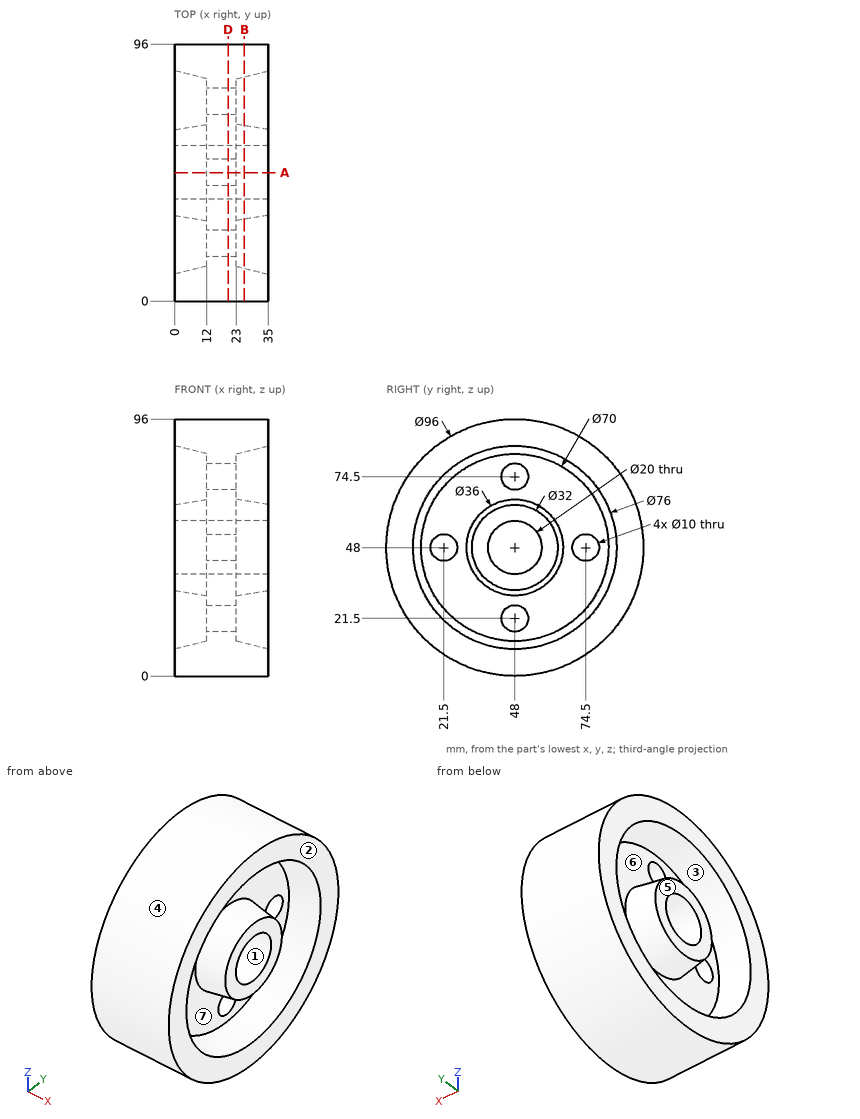
Input: dimensioned drawing with shaded views. Units: mm. Origin: part minimum x, y, z. A direction names the side the tool comes from. Coordinates: 2 decimals unless noted, no trailing zeros. Write each loop counter-clockwise with the first axis right and the second up, starting at its lowest first coordinate (ties: lowest second). Pieces come first, ordered by that corner, then holes. Notation, with made-up numbers: (30, -32) -> (84, -32) arc R22 ccw to (84, -4) -> close; hole circle Ø10 at (50, 29). An arc over 180 degrees is marked (long way). Return JSON: item names as keys, results as strings. Group by question number.
1) Ray query, line 1 along Y through (x, z) = (19, 48); line 2 along Z through (x, y) = (33, 52); line 3 along Z through (x, y) = (29, 46). Return the intervals inside material, ascending.
2) Section query D-D, the plane x = 20. Return loops of the section in (y, z).
3) Mould query, pull axis Y, two halves, no side actions, for the marked faces 1, 2, 3 and 4. Classes: +Y half, -Y half, draft (parallel to the pull), parting line (faces both ways), or undercut.
4) Section query A-A, the plane y = 48. State how many separate pieces and enclosed holes the cut face has, plus the area to 3 significant figures.
5) Contact query for flat-ended pins moving along their axis: P1, Ø1.5, axis at y = 45.5, z = 72, coming from the -X side; P2, Ø12, axis at x = 9.5, z = 65.5, coming from the +Y side; P3, Ø11.5, axis at y = 21.5, z = 48, coming from the -X side; P4, Ø13, axis at y = 48, z = 21.5, coming from the +X side. Output: stop coordinate, or through.
6) Set-up query: the marked faces 5, 6 and 7. Return all of +Z, -Z, +X, -X, +Y, -Y with unobstructed straight access to the full face (end or side cutting, diameter ignored); none if empty.
7) Section query B-B, the plane x = 26. Return loops of the section in (y, z).
From the geometry:
{
 "1": {"line 1": "0 to 16.5, 26.5 to 38, 58 to 69.5, 79.5 to 96", "line 2": "0.17 to 10.71, 32.16 to 38.83, 57.17 to 63.84, 85.29 to 95.83", "line 3": "0.04 to 11.55, 31.12 to 38.2, 57.8 to 64.88, 84.45 to 95.96"},
 "2": {"outline": "circle Ø96 at (48, 48); hole circle Ø10 at (21.5, 48); hole circle Ø20 at (48, 48); hole circle Ø10 at (48, 21.5); hole circle Ø10 at (48, 74.5); hole circle Ø10 at (74.5, 48)"},
 "3": {"face 1": "undercut", "face 2": "draft", "face 3": "undercut", "face 4": "parting line"},
 "4": {"separate pieces": "4", "enclosed holes": "0", "area": "1,500 mm²"},
 "5": {"P1": "through", "P2": "y = 94.6", "P3": "x = 12", "P4": "x = 23"},
 "6": {"face 5": "+Z, -Z, -X, +Y, -Y", "face 6": "-X", "face 7": "+X"},
 "7": {"outline": "circle Ø96 at (48, 48); circle Ø35 at (48, 48); hole circle Ø71.5 at (48, 48); hole circle Ø20 at (48, 48)"}
}
